Check sheet for the drawn part. Datum: minimum x, y, z corner. Units: mm. A direction names the side the tool comes from. Give positions to 0.01 mm unless a question says otherwise; leave off trailing zeros. Write each loop counter-clockwise with the first axis right and the second up, starting at its lowest first coordinate (ties: lowest second). Pieces come first, ordered by that corner, then holes.
(1) Cross-section at D-D (y = 4.25). Record the boundary of the cut face in (x, z).
(2) Cross-section at C-C (z = 2.25). Record the boundary of the cut face in (x, y).
(3) Cross-section at A-A (x = 5). Record the boundary of the cut face in (y, z), and give its area (3 significant figures).
(4) Cross-section at B-B (y = 1.25). Record the boundary of the cut face in (x, z).
(5) Tool access check on the marked faces 1, 2 and 3. Record the directions out of +Z, -Z, +X, -X, +Y, -Y that give a thin tool (end or side, any length) a straight path to the whole face; none if there is none.
(6) Depth check by flat-ended pin: P1, Ø2.5, axis at x = 6, z = 3, coming from the +Y side; P2, Ø0.8, axis at y = 3.5, z = 3, coming from the -X side; P3, Ø1.1, axis at y = 3.5, z = 2, coming from the +X side. Enter the tip coordinate at first touch or a pass-through.
(7) Thickness scan on line 1 along Z through (x, y) = (3.5, 1.75); line 2 along X through (y, z) = (6, 18) (3 decimals); line 3 along X through (y, z) = (6, 25.5). Record the ranges inside material, lowest first.
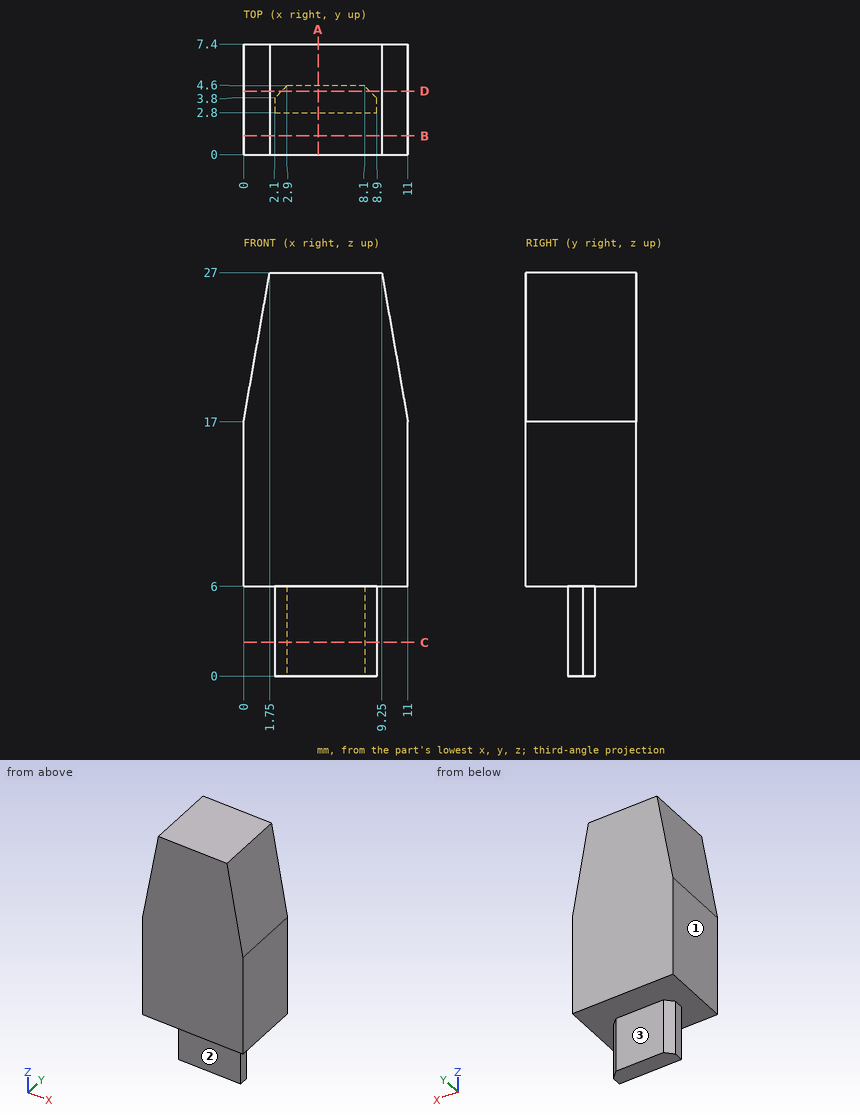
Reply:
1. outline: (0, 6) - (2.55, 6) - (2.55, 0) - (8.45, 0) - (8.45, 6) - (11, 6) - (11, 17) - (9.25, 27) - (1.75, 27) - (0, 17) - close
2. outline: (2.1, 2.8) - (8.9, 2.8) - (8.9, 3.8) - (8.1, 4.6) - (2.9, 4.6) - (2.1, 3.8) - close
3. outline: (0, 6) - (2.8, 6) - (2.8, 0) - (4.6, 0) - (4.6, 6) - (7.4, 6) - (7.4, 27) - (0, 27) - close
3. area: 166 mm2
4. outline: (0, 6) - (11, 6) - (11, 17) - (9.25, 27) - (1.75, 27) - (0, 17) - close
5. face 1: +Z, -Z, -X, +Y, -Y
5. face 2: -Z, +X, -X, -Y
5. face 3: -Z, +X, -X, +Y
6. P1: stops at y = 4.6
6. P2: stops at x = 2.1
6. P3: stops at x = 8.9
7. line 1: z = 6 to 27
7. line 2: x = 0.175 to 10.825
7. line 3: x = 1.49 to 9.51
